Could you check a few things on this model? Use its own coordinates, in mm. Face numbers are marked on the shaded views. A direction names the side the tool comes from. Round coordinates to 2 decimals unless told otherwise and drop trailing zeros. Loops run counter-clockwise (first coordinate to the right, second up) from the corner with the lowest first, then second, coordinate; pieces in that order, holes last. Notation, with made-up numbers: (36, 75) -> (74, 75) arc R30 cw to (74, 101) -> close; hole circle Ø7 at (62.5, -29). An arc over 180 degrees is marked (long way). Put each result on its own line as item: value. Start each with the question number.
1. I need wall thicknesses on line 1 (X direction, y = -38, z = 32); line 2 (Z direction, x = 16.5, y = -34.5); line 3 (Z direction, x = 56, y = -19). Which ranges of each line are inside material? Lowest first, please. Write a range as [from, to].
2. Imagine slicing it at D-D, the plane y = -22.5. Please give me the cut outline in (x, z).
3. I'm going to push flat-ended pins straight in: P1, Ø14, axis at y = -43.5, z = 47, coming from the +X side; P2, Ø10, axis at x = 131.5, y = -25.5, coming from the +Z side; P3, Ø15, axis at x = 38.5, y = -30.5, coming from the +Z side. Where does each tip first touch, or does it pass through?
4. If we mould it in two halves opening along Y, with no side actions, what happens to the marked faces 6, 7 and 8? For each: pulls with the +Y half, pulls with the -Y half, needs draft (parallel to the pull), parting line crosses it, or undercut.
5. Imagine slicing it at B-B, the plane x = 19.5. Please give me the cut outline in (y, z).
6. Which directions (+Z, -Z, +X, -X, +Y, -Y) give clear straight access to the entire face, cutting with the end or side of a thin tool? Please do the marked faces 1, 2, 3, 4 and 5.
7. Imagine slicing it at C-C, the plane y = -67.5. Please give me the cut outline in (x, z), and give its area (3 significant figures).
8. Imagine slicing it at A-A, the plane z = 43. Please give me the cut outline in (x, y).
```python
from build123d import *

# Parameters (mm, degrees)
F1_DEPTH = 76.2
F4_DEPTH = 187.96


with BuildPart() as f1:
    # F0 (on Front) → F1 (new body)
    with BuildSketch(Plane.XZ):
        Polygon((0, 50.8), (0, 0), (152.4, 0), (152.4, 38.1), (82.55, 38.1), (76.2, 50.8), (50.8, 50.8), (50.8, 38.1), (63.5, 38.1), (63.5, 25.4), (12.7, 25.4), (12.7, 38.1), (25.4, 38.1), (25.4, 50.8), align=None)
    extrude(amount=F1_DEPTH)

    # F3 (on offset) → F4 (cut)
    with BuildSketch(Plane(origin=(-25.4, 0, 0), x_dir=(0, -1, 0), z_dir=(-1, 0, 0))):
        Polygon((63.5, 8.429470472), (12.7, 8.429470472), (25.4, 0), (50.8, 0), align=None)
    extrude(amount=-F4_DEPTH, mode=Mode.SUBTRACT)


solid = f1.part
```
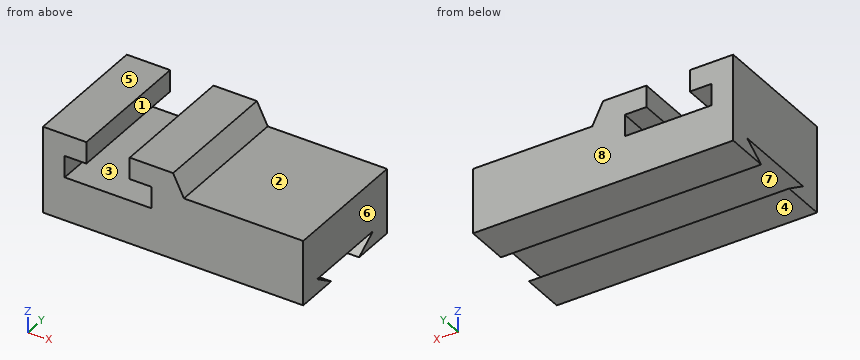
Entries:
1. line 1: [0, 12.7], [63.5, 152.4]
1. line 2: [8.43, 25.4], [38.1, 50.8]
1. line 3: [0, 4.25], [8.43, 25.4], [38.1, 50.8]
2. outline: (0, 0) -> (152.4, 0) -> (152.4, 1.92) -> (0, 1.92) -> close; (0, 8.43) -> (152.4, 8.43) -> (152.4, 38.1) -> (82.55, 38.1) -> (76.2, 50.8) -> (50.8, 50.8) -> (50.8, 38.1) -> (63.5, 38.1) -> (63.5, 25.4) -> (12.7, 25.4) -> (12.7, 38.1) -> (25.4, 38.1) -> (25.4, 50.8) -> (0, 50.8) -> close
3. P1: x = 81.6
3. P2: z = 38.1
3. P3: z = 25.4
4. face 6: needs draft
4. face 7: undercut
4. face 8: pulls with the +Y half
5. outline: (-76.2, 0) -> (-50.8, 0) -> (-63.5, 8.43) -> (-12.7, 8.43) -> (-25.4, 0) -> (0, 0) -> (0, 25.4) -> (-76.2, 25.4) -> close; (-76.2, 38.1) -> (0, 38.1) -> (0, 50.8) -> (-76.2, 50.8) -> close
6. face 1: +Z, +Y, -Y
6. face 2: +Z, +X, +Y, -Y
6. face 3: +Y, -Y
6. face 4: -Z, +X, -X, +Y, -Y
6. face 5: +Z, +X, -X, +Y, -Y
7. outline: (0, 0) -> (152.4, 0) -> (152.4, 38.1) -> (82.55, 38.1) -> (76.2, 50.8) -> (50.8, 50.8) -> (50.8, 38.1) -> (63.5, 38.1) -> (63.5, 25.4) -> (12.7, 25.4) -> (12.7, 38.1) -> (25.4, 38.1) -> (25.4, 50.8) -> (0, 50.8) -> close
7. area: 5,850 mm^2
8. outline: (0, -76.2) -> (25.4, -76.2) -> (25.4, 0) -> (0, 0) -> close; (50.8, -76.2) -> (80.1, -76.2) -> (80.1, 0) -> (50.8, 0) -> close
